from build123d import *

# Parameters (mm, degrees)
F0_W           = 241
F0_H           = 43.5
F1_DEPTH       = 10
F2_SIZE        = 3
F4_DEPTH       = 2
F6_D           = 5
F6_CSINK_D     = 8.96
F6_CSINK_ANGLE = 90


with BuildPart() as f1:
    # F0 (on Front) → F1 (new body)
    with BuildSketch(Plane.XZ):
        with Locations((120.5, 21.75)):
            Rectangle(F0_W, F0_H)
    extrude(amount=F1_DEPTH)

    # F2
    f2_edges = [f1.edges().sort_by_distance(p)[0] for p in [
        (241, -5, 43.5),
        (241, -5, 0),
        (0, -5, 43.5),
        (0, -5, 0),
    ]]
    chamfer(f2_edges, length=F2_SIZE)

    # F3 (on face) → F4 (join)
    with BuildSketch(Plane(origin=(0, 0, 0), x_dir=(-1, 0, 0), z_dir=(0, 1, 0))):
        Polygon((-9.4982709692, 33.0000003319), (-9.4999992993, 37.5), (-231.4982709692, 37.5), (-231.4982709692, 33.0000003319), align=None)
    extrude(amount=F4_DEPTH)

    # F6 (through all)
    with Locations(Plane.XZ.offset(10)):
        with Locations((236.5, 35.5), (236.5, 8), (4.5, 35.5), (4.5, 8)):
            CounterSinkHole(F6_D / 2, F6_CSINK_D / 2, counter_sink_angle=F6_CSINK_ANGLE)


solid = f1.part
Can you work these out from the model? Positions are in its coordinate system, mm. Give positions to 0.01 mm unless a question says otherwise; leave off trailing zeros. Order: outer loops, then holes, each group sorted by start corner. A loop starts at its lowest first (then second) coordinate and runs counter-clockwise, first axis right, second up. Notation, with made-up numbers: M 78,39 L 118,39 A8 ccw 118,48 Z; hole C -4.75,-10.5 d8. An arc over 180 degrees is marked long. One line per item, written item: value.
Item 1: For pin 1 (1 mm diameter, centred on x = 139.5, y = 1, fed in from +Z); pin 2 (6 mm diameter, centred on x = 4.5, z = 8, fed in from -Y); pin 3 (1 mm diameter, centred on x = 84.5, z = 7.5, fed in from +Y); pin 4 (4.5 mm diameter, centred on x = 236.5, z = 8, fed in from +Y), each with a flat end and sliding along its axis, tell me the tip position at first contact or that it passes through.
Verdict:
pin 1: z = 37.5
pin 2: y = -8.52
pin 3: y = 0
pin 4: through
Item 2: If we section it at A-A on z = 8: State how many separate pieces and enclosed holes the cut face has, and give its area (3 significant figures).
Verdict:
separate pieces: 3
enclosed holes: 0
area: 2,300 mm2
Item 3: If we section it at B-B on x = 114: Write out the boundary of the cut face in (y, z), and give its area (3 significant figures).
Verdict:
outline: M -10,0 L 0,0 L 0,33 L 2,33 L 2,37.5 L 0,37.5 L 0,43.5 L -10,43.5 Z
area: 444 mm2
Item 4: If we section it at D-D on z = 19.5: Write out the boundary of the cut face in (x, y).
Verdict:
outline: M 0,-10 L 241,-10 L 241,0 L 0,0 Z
Item 5: Please list where these lines run through material, in increasing order: line 1 (Z direction, x = 4.5, y = -1.75); line 2 (X direction, y = -3, z = 35.5); line 3 (X direction, y = -2.5, z = 10).
Verdict:
line 1: 0 to 5.5, 10.5 to 33, 38 to 43.5
line 2: 0 to 2, 7 to 234, 239 to 241
line 3: 0 to 3, 6 to 235, 238 to 241
Item 6: If we mould it in two halves opening along X, with no side actions, what happens to faces 1 (the face through (119, -10, 22)), 2 (the face through (241, -5, 21)), 3 (the face through (234.19, -3.95, 7.04))? For each: pulls with the +X half, pulls with the -X half, needs draft (parallel to the pull), parting line crosses it, or undercut.
Verdict:
face 1: needs draft
face 2: pulls with the +X half
face 3: undercut
